from build123d import *

# Parameters (mm, degrees)
BOSS_EXTRUDE1_DEPTH     = 33.274
SKETCH3_R               = 6.349999999999995
SKETCH3_R_2             = 6.349999999999994
SKETCH3_R_3             = 6.349999999999996
CUT_EXTRUDE1_DEPTH      = 131.05221672851255
BOSS_EXTRUDE2_DEPTH     = 20.574
SKETCH5_R               = 2.0193000000000074
SKETCH5_R_2             = 2.0193000000000025
CUT_EXTRUDE2_DEPTH      = 134.57623111628357
CUT_EXTRUDE3_REACH      = 109.787
CUT_EXTRUDE3_END_RADIUS = 41.90999999999999
SKETCH6_R               = 3.1750000000000003
FILLET1_R               = 3.175
FILLET2_R               = 1.9176999999999997
FILLET3_R               = 1


with BuildPart() as part:
    # Sketch1 → Boss-Extrude1 (new body)
    with BuildSketch(Plane(origin=(0, 0, 0), x_dir=(1, 0, 0), z_dir=(0, 1, 0))):
        with BuildLine():
            Line((0, 0), (33.655, 6.94e-15))
            Line((33.655, 6.94e-15), (33.655, 3.954122740703593))
            ThreePointArc((33.655, 3.954122740703593), (11.216985165351097, 18.91541903613836), (2.5400000000000076, 44.449999999999704))
            Line((2.5400000000000076, 44.449999999999704), (2.540000000000145, 80.00999999999985))
            Line((2.540000000000145, 80.00999999999985), (8.890000000000144, 80.00999999999985))
            Line((8.890000000000144, 80.00999999999985), (8.890000000000148, 86.36))
            Line((8.890000000000148, 86.36), (44.449999999999854, 86.35999999999999))
            ThreePointArc((44.449999999999854, 86.35999999999999), (69.98458096386148, 77.68301483464901), (84.9458772592964, 55.244999999999976))
            Line((84.9458772592964, 55.244999999999976), (88.89999999999999, 55.245))
            Line((88.89999999999999, 55.245), (88.89999999999999, 88.89999999999999))
            Line((88.89999999999999, 88.89999999999999), (0, 88.89999999999999))
            Line((0, 88.89999999999999), (0, 0))
        make_face()
    extrude(amount=BOSS_EXTRUDE1_DEPTH)

    # Sketch3 → Cut-Extrude1 (cut, through all)
    with BuildSketch(Plane(origin=(0, 33.274, 0), x_dir=(1, 0, 0), z_dir=(0, 1, 0))):
        with Locations((9.525000000000004, 79.37499999999999)):
            Circle(SKETCH3_R)
        with Locations(Location((79.375, 79.37499999999999, 0), (0, 0, 270))):
            Circle(SKETCH3_R_2)
        with Locations(Location((9.525000000000006, 9.524999999999991, 0), (0, 0, 270))):
            Circle(SKETCH3_R_3)
    extrude(amount=-CUT_EXTRUDE1_DEPTH, mode=Mode.SUBTRACT)

    # Sketch4 → Boss-Extrude2 (add)
    with BuildSketch(Plane.XZ):
        with BuildLine():
            Line((33.655, -6.94e-15), (33.65499999999999, -3.9541227407036))
            ThreePointArc((33.65499999999999, -3.9541227407036), (44.66502117576741, -2.5405515916282795), (55.65995813673013, -4.067021672829062))
            ThreePointArc((55.65995813673013, -4.067021672829062), (58.23891440878839, -3.8021336224280984), (59.95265305936133, -1.8568107777654739))
            Line((59.95265305936133, -1.8568107777654739), (60.12692723379523, -1.3779964187142884))
            ThreePointArc((60.12692723379523, -1.3779964187142884), (59.94763198470919, 1.464665073241983), (57.73949808555085, 3.263835945500561))
            ThreePointArc((57.73949808555085, 3.263835945500561), (49.009557209614336, 4.869685096848045), (40.13317606170841, 4.89152339648416))
            add(Edge.make_bspline(
                [(33.655, -6.94e-15), (36.19500000000001, -6.94e-15), (36.75939668417103, 4.596355947712086), (40.13317606170841, 4.89152339648416)],
                knots=[0, 0, 0, 0, 1, 1, 1, 1], degree=3))
        make_face()
        with BuildLine():
            Line((87.04318922223452, -28.94734694063866), (87.52200358128572, -28.77307276620477))
            ThreePointArc((87.52200358128572, -28.77307276620477), (90.364665073242, -28.952368015290805), (92.16383594550055, -31.160501914449153))
            ThreePointArc((92.16383594550055, -31.160501914449153), (93.76968509684802, -39.89044279038568), (93.79152339648414, -48.7668239382916))
            add(Edge.make_bspline(
                [(88.89999999999999, -55.245), (88.89999999999999, -52.705), (93.49635594771208, -52.140603315828955), (93.79152339648414, -48.7668239382916)],
                knots=[0, 0, 0, 0, 1, 1, 1, 1], degree=3))
            Line((88.89999999999999, -55.245), (84.9458772592964, -55.245))
            ThreePointArc((84.9458772592964, -55.245), (86.35944840837172, -44.23497882423258), (84.83297832717093, -33.240041863269866))
            ThreePointArc((84.83297832717093, -33.240041863269866), (85.09786637757189, -30.661085591211602), (87.04318922223452, -28.94734694063866))
        make_face()
    extrude(amount=-BOSS_EXTRUDE2_DEPTH)

    # Sketch5 → Cut-Extrude2 (cut, through all)
    with BuildSketch(Plane(origin=(0, 33.274, 0), x_dir=(1, 0, 0), z_dir=(0, 1, 0))):
        with Locations(Location((85.725, 66.03999999999999, 0), (0, 0, 270))):
            Circle(SKETCH5_R)
        with Locations(Location((22.860000000000007, 3.174999999999997, 0), (0, 0, 270))):
            Circle(SKETCH5_R_2)
    extrude(amount=-CUT_EXTRUDE2_DEPTH, mode=Mode.SUBTRACT)

    # Cut-Extrude3: up to this cylinder (the profile starts outside it)
    cut_extrude3_end = Plane(origin=(44.449999999999996, 3.8099999999999987, -44.449999999999996), z_dir=(0, -1, 0)) * Cylinder(CUT_EXTRUDE3_END_RADIUS, 304.394, mode=Mode.PRIVATE)
    # Sketch6 → Cut-Extrude3 (cut, up to the surface)
    with BuildSketch(Plane(origin=(49.00955720961435, 20.573999999999995, 4.869685096848044), x_dir=(0.9957537875398352, 0, -0.0920564750578304), z_dir=(0.0920564750578304, 0, 0.9957537875398352)), mode=Mode.PRIVATE) as cut_extrude3_sk1:
        with Locations((0, -16.763999999999996)):
            Circle(SKETCH6_R)
    cut_extrude3_tool1 = extrude(cut_extrude3_sk1.sketch, amount=-CUT_EXTRUDE3_REACH, mode=Mode.PRIVATE) - cut_extrude3_end
    cut_extrude3 = cut_extrude3_tool1.solids().sort_by_distance((49.009557, 3.81, 4.869685))[0]
    add(cut_extrude3, mode=Mode.SUBTRACT)

    # Mirror1: Cut-Extrude3 across plane
    add(cut_extrude3.mirror(Plane(origin=(44.449999999999996, 0, -44.449999999999996), x_dir=(0.7071067811865477, 0, 0.7071067811865474), z_dir=(-0.7071067811865476, 0, 0.7071067811865476))), mode=Mode.SUBTRACT)

    # Fillet1
    fillet1_edges = [part.edges().sort_by_distance(p)[0] for p in [
        (0, 16.637, -88.89999999999999),
    ]]
    fillet(fillet1_edges, radius=FILLET1_R)

    # Fillet2
    fillet2_edges = [part.edges().sort_by_distance(p)[0] for p in [
        (33.655, 26.924, -3.9541227407035944),
        (33.655, 26.924, -6.94e-15),
        (88.89999999999999, 26.924, -55.245),
        (84.9458772592964, 26.924, -55.244999999999976),
    ]]
    fillet(fillet2_edges, radius=FILLET2_R)

    # Fillet3
    fillet3_edges = [part.edges().sort_by_distance(p)[0] for p in [
        (88.89999999999999, 16.637, -88.89999999999999),
        (0, 16.637, 0),
    ]]
    fillet(fillet3_edges, radius=FILLET3_R)


solid = part.part
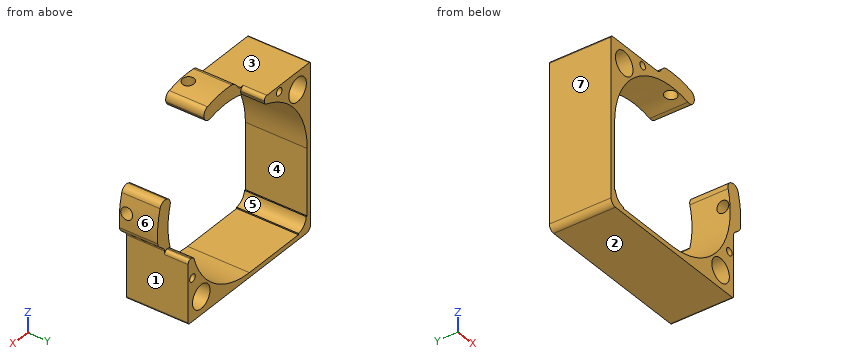
The model under review builds one solid part; all positions refer to its coordinate system, in mm. Face numbers are marked on the shaded views. A direction names the side the tool comes from. Give positions to 0.01 mm unless a question says otherwise; leave off trailing zeros. Loops run counter-clockwise (first coordinate to the right, second up) from the corner with the lowest first, then second, coordinate; pieces in that order, holes last. Notation, with made-up numbers: (13, 13) -> (55, 13) arc R10 cw to (55, 32) -> close; hole circle Ø2 at (23, -30). An arc over 180 degrees is marked (long way). Put each result on its own line as item: value. Start each with the question number.
1. Clearance check with flat-ended pins moving along their axes: P1, Ø12, axis at x = 27.5, z = -15.5, coming from the -Y side; P2, Ø0.5, axis at y = 27.5, z = -2.5, coming from the +X side (3 decimals); P3, Ø0.5, axis at x = 86.5, y = 25, coming from the +Z side (3 decimals); P4, Ø0.5, axis at x = 3, y = 10, coming from the +Z side. State where each tip first meets the part, or that it passes through.
2. Mouldability with a two-part tool opening along Z and no side actions: class the marked faces 5, 6 and 7 as released by +Z, released by -Z, zero draft, split by the parting line, or undercut.
3. For the marked faces 1, 2, 3 and 4, list the 3-axis set-ups (+Z, -Z, +X, -X, +Y, -Y) from which the entire face can be reached by the end or side of a thin tool; tool diameter is ignored.
4. We need section A-A on z = -7.5. State the section outline as (x, y) points, then the cut area to 3 significant figures.
5. We need section D-D on y = 28. State the section outline as (x, z) points (3 decimals), then the cut area to 3 significant figures.
6. We need section C-C on z = -66.04. State the section outline as (x, y) points, then the cut area to 3 significant figures.
7. Wall thickness on probe 1 along Z at (x, y) = (37.5, 22); probe 2 along Z at (x, y) = (34, 2); probe 3 along Z at (x, y) = (76, 16): over which ranges is each line inside the solid? List them lowest first.
8. We need section B-B on x = 22.86. State the section outline as (y, z) points.
Determined:
1. P1: through
1. P2: x = 33.655
1. P3: z = -55.245
1. P4: z = 0
2. face 5: undercut
2. face 6: split by the parting line
2. face 7: zero draft
3. face 1: -Z, +X, +Y, -Y
3. face 2: -Z, +X, -X, +Y, -Y
3. face 3: +Z, -X, +Y, -Y
3. face 4: +Y, -Y
4. outline: (0, 0) -> (3.51, 0) -> (3.51, 33.27) -> (0, 33.27) -> close; (15.54, 0) -> (24.67, 0) -> (24.67, 33.27) -> (15.54, 33.27) -> close
4. area: 420 mm^2
5. outline: (0, -85.725) arc R3.175 ccw to (3.175, -88.9) -> (87.9, -88.9) arc R1 ccw to (88.9, -87.9) -> (88.9, -57.163) arc R1.918 ccw to (86.982, -55.245) -> (86.393, -55.245) arc R1.918 ccw to (84.558, -56.606) arc R41.91 cw to (44.45, -86.36) -> (8.89, -86.36) -> (8.89, -85.693) arc R6.35 cw to (3.207, -80.01) -> (2.54, -80.01) -> (2.54, -44.45) arc R41.91 cw to (32.294, -4.342) arc R1.918 ccw to (33.655, -2.507) -> (33.655, -1.918) arc R1.918 ccw to (31.737, 0) -> (1, 0) arc R1 ccw to (0, -1) -> close; hole circle Ø12.7 at (9.525, -9.525); hole circle Ø4.039 at (22.86, -3.175); hole circle Ø12.7 at (79.375, -79.375); hole circle Ø4.039 at (85.725, -66.04)
5. area: 1,080 mm^2
6. outline: (0, 0) -> (2.54, 0) -> (2.54, 33.27) -> (0, 33.27) -> close; (80.37, 0) -> (83.71, 0) -> (83.71, 33.27) -> (80.37, 33.27) -> close; (87.74, 0) -> (88.9, 0) -> (88.9, 33.27) -> (87.74, 33.27) -> close
6. area: 234 mm^2
7. probe 1: -88.9 to -86.36
7. probe 2: -88.9 to -86.36, -3.86 to 0.03
7. probe 3: -88.9 to -84.75, -74 to -72.04
8. outline: (0, -88.9) -> (33.27, -88.9) -> (33.27, -86.36) -> (0, -86.36) -> close; (0, -8.53) -> (33.27, -8.53) -> (33.27, -5.19) -> (0, -5.19) -> close; (0, -1.16) -> (33.27, -1.16) -> (33.27, 0) -> (0, 0) -> close
